from build123d import *

# Parameters (mm, degrees)
SKETCH7_R           = 5
BOSS_EXTRUDE1_DEPTH = 90
SKETCH8_R           = 7.447394551
CUT_EXTRUDE1_DEPTH  = 90
FILLET1_R           = 15


with BuildPart() as part:
    # Sketch7 → Boss-Extrude1 (new body)
    with BuildSketch(Plane(origin=(0, 0, 0), x_dir=(1, 0, 0), z_dir=(0, 1, 0))):
        with BuildLine():
            Line((7.357897338, -3.140278136), (19.375959063, 25.018904128))
            ThreePointArc((19.375959063, 25.018904128), (21.522528234, 27.403649264), (24.679857301, 27.974649904))
            Line((24.679857301, 27.974649904), (102, 27.974649904))
            ThreePointArc((102, 27.974649904), (111.729786481, 29.518933772), (120.503246637, 34))
            Line((120.503246637, 34), (242, 34))
            Line((242, 34), (242, 37))
            Line((242, 37), (119.499086706, 37))
            ThreePointArc((119.499086706, 37), (111.253686824, 32.523169315), (102, 30.974649904))
            Line((102, 30.974649904), (24.879394183, 30.974649904))
            ThreePointArc((24.879394183, 30.974649904), (19.95222913, 29.961796073), (16.616747562, 26.196508428))
            Line((16.616747562, 26.196508428), (7.05006467, 3.781082934))
            ThreePointArc((7.05006467, 3.781082934), (-7.992099353, -0.355454547), (7.357897338, -3.140278136))
        make_face()
        with Locations(Location((0, 0, 0), (0, 0, 90))):
            Circle(SKETCH7_R, mode=Mode.SUBTRACT)
    extrude(amount=BOSS_EXTRUDE1_DEPTH)

    # Sketch8 → Cut-Extrude1 (cut)
    with BuildSketch(Plane.XY.offset(-34)):
        with Locations((140.503246637, 75)):
            Circle(SKETCH8_R)
        with Locations((140.503246637, 15)):
            Circle(SKETCH8_R)
        with Locations((222, 75)):
            Circle(SKETCH8_R)
        with Locations((222, 15)):
            Circle(SKETCH8_R)
    extrude(amount=-CUT_EXTRUDE1_DEPTH, mode=Mode.SUBTRACT)

    # Fillet1
    fillet1_edges = [part.edges().sort_by_distance(p)[0] for p in [
        (242, 0, -35.5),
        (242, 90, -35.5),
    ]]
    fillet(fillet1_edges, radius=FILLET1_R)


solid = part.part
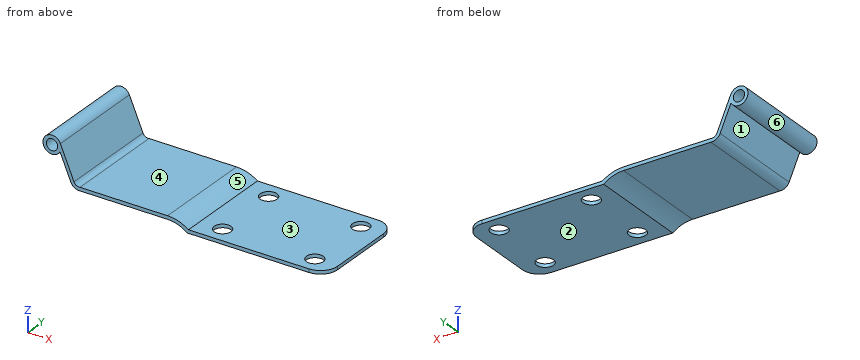
Build history of the part. All positions in model axes, mm. Face numbers are marked on the shaded views. A direction names the side the tool comes from. Round coordinates to 2 decimals unless told otherwise and drop trailing zeros. Order: outer loops, then holes, each group sorted by start corner. A loop starts at its lowest first (then second) coordinate and runs counter-clockwise, first axis right, second up. Notation, with made-up numbers: M -31.75,63 L -0.75,63 A34 cw -0.75,93 Z; hole C -5,83 d11. An arc over 180 degrees is marked long. Use CSV: the item, a comma, the result in double quotes. Start each with the question number.
(1) Cut at B-B on y = 47. List the corners of the cut face in (x, z), then the cut area to 3 significant figures.
(2) Cut at C-C on z = 0. List the corners of the cut face in (x, y), then the cut area to 3 significant figures.
(3) Flat gauge pins, fed straight in: P1, Ø17, axis at x = 222, y = 15, coming from the +Z side; P2, Ø23, axis at x = 61, y = 67, coming from the -Z side; P3, Ø5, axis at y = 29.5, z = -29, coming from the -X side; P4, Ø24, axis at x = 140.5, y = 15, coming from the -Z side. Where does each tip first touch, or does it go through?
(4) Drill centre lines: probe 1 along Y at (x, z) = (222, -35.9); probe 2 along X at (y, z) = (77, -34.5); probe 3 along Z at (x, y) = (202.5, 48). Where is each one in solid material? Low to high.
(5) Cut at D-D on y = 20. List the corners of the cut face in (x, z).
(6) Cut at A-A on x = 222. List the corners of the cut face in (y, z), then the cut area to 3 significant figures.
(7) Tool access for the marked faces 1, 2 and 3: list every direction of +Z, -Z, +X, -X, +Y, -Y with a clear straight run to the whole face (end or side of a thin tool).
(8) Mould opens along X. For the marked faces 4, 5 and 6 say: +X half, -X half, draft (parallel to the pull), parting line (faces both ways), or undercut.
Findings:
1,outline,"M 7.05,-3.78 L 16.62,-26.2 A7.96 ccw 24.88,-30.97 L 102,-30.97 A28.42 cw 119.5,-37 L 242,-37 L 242,-34 L 120.5,-34 A31.42 ccw 102,-27.97 L 24.68,-27.97 A4.96 cw 19.38,-25.02 L 7.36,3.14 A8 ccw long Z; hole C 0,0 d10"
1,area,"882 mm^2"
2,outline,"M -8,0 L -5,0 L -5,90 L -8,90 Z; M 5,0 L 8.7,0 L 8.7,90 L 5,90 Z"
2,area,"603 mm^2"
3,P1,"stops at z = -34"
3,P2,"stops at z = -30.97"
3,P3,"stops at x = 16.75"
3,P4,"stops at z = -37"
4,probe 1,"y = 0 to 7.55, 22.45 to 67.55, 82.45 to 90"
4,probe 2,"x = 115.71 to 133.33, 147.68 to 214.83, 229.17 to 241.87"
4,probe 3,"z = -37 to -34"
5,outline,"M 7.05,-3.78 L 16.62,-26.2 A7.96 ccw 24.88,-30.97 L 102,-30.97 A28.42 cw 119.5,-37 L 134.98,-37 L 134.98,-34 L 120.5,-34 A31.42 ccw 102,-27.97 L 24.68,-27.97 A4.96 cw 19.38,-25.02 L 7.36,3.14 A8 ccw long Z; M 146.02,-37 L 216.48,-37 L 216.48,-34 L 146.02,-34 Z; M 227.52,-37 L 242,-37 L 242,-34 L 227.52,-34 Z; hole C 0,0 d10"
6,outline,"M 0,-37 L 7.55,-37 L 7.55,-34 L 0,-34 Z; M 22.45,-37 L 67.55,-37 L 67.55,-34 L 22.45,-34 Z; M 82.45,-37 L 90,-37 L 90,-34 L 82.45,-34 Z"
6,area,"181 mm^2"
7,face 1,"-Z, +Y, -Y"
7,face 2,"-Z, +X, -X, +Y, -Y"
7,face 3,"+Z, +X, +Y, -Y"
8,face 4,"draft"
8,face 5,"+X half"
8,face 6,"undercut"
